Input: part model. Units: mm. Frame: model coordinates. Face numbers are marked on the shaded views. A direction names the side the tool comes from. Give positions to 0.01 mm unless a question says otherwise; leave off trailing zeros. Order: outer loops, then holes, each group sorted by start corner. A loop starts at its lowest first (then second) coordinate and runs counter-clockwise, first axis right, second up. Notation, with made-up numbers: M 67,74 L 109,74 A15 cw 109,101 Z; hole C -22.5,-15.75 d10. An arc over 180 degrees is marked long. Use a Markdown table: item, result.
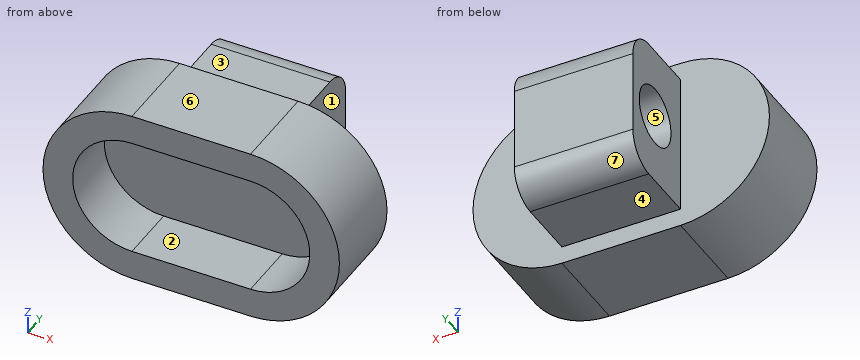
from build123d import *

# Parameters (mm, degrees)
F1_DEPTH = 15
F3_DEPTH = 5
F4_W     = 20
F4_H     = 24
F5_DEPTH = 15
F6_R     = 5
F7_R     = 5
F8_DEPTH = 25


with BuildPart() as f1:
    # F0 (on Front) → F1 (new body)
    with BuildSketch(Plane.XZ):
        with BuildLine():
            Line((-10, -15), (10, -15))
            ThreePointArc((10, -15), (25, 0), (10, 15))
            Line((10, 15), (-10, 15))
            ThreePointArc((-10, 15), (-25, 0), (-10, -15))
        make_face()
        with BuildLine():
            ThreePointArc((-10, -10), (-20, 0), (-10, 10))
            Line((-10, 10), (10, 10))
            ThreePointArc((10, 10), (20, 0), (10, -10))
            Line((10, -10), (-10, -10))
        make_face(mode=Mode.SUBTRACT)
    extrude(amount=F1_DEPTH)

    # F2 (on face) → F3 (join)
    with BuildSketch(Plane(origin=(0, 0, 0), x_dir=(-1, 0, 0), z_dir=(0, 1, 0))):
        with BuildLine():
            ThreePointArc((10, -10), (20, 0), (10, 10))
            Line((10, 10), (-10, 10))
            ThreePointArc((-10, 10), (-20, 0), (-10, -10))
            Line((-10, -10), (10, -10))
        make_face()
    extrude(amount=-F3_DEPTH)

    # F4 (on face) → F5 (join)
    with BuildSketch(Plane(origin=(0, 0, 0), x_dir=(-1, 0, 0), z_dir=(0, 1, 0))):
        Rectangle(F4_W, F4_H)
    extrude(amount=F5_DEPTH)

    # F6
    f6_edges = [f1.edges().sort_by_distance(p)[0] for p in [
        (0, 15, -12),
        (0, 15, 12),
    ]]
    fillet(f6_edges, radius=F6_R)

    # F7 (on face) → F8 (cut)
    with BuildSketch(Plane.YZ.offset(10)):
        with Locations((8, 0)):
            Circle(F7_R)
    extrude(amount=-F8_DEPTH, mode=Mode.SUBTRACT)


solid = f1.part
1) Cut plane D-D on x = 11.5. Return loops of the section in (y, z), and give its area (3 significant figures).
Response values:
| item | result |
|---|---|
| outline | M -15,-14.92 L 0,-14.92 L 0,14.92 L -15,14.92 L -15,9.89 L -5,9.89 L -5,-9.89 L -15,-9.89 Z |
| area | 250 mm² |
2) Mould query, pull axis Y, two halves, no side actions, for the marked faces 5, 6 and 7. Classes: released by +Y, released by -Y, zero draft, split by the parting line, or undercut.
Response values:
| item | result |
|---|---|
| face 5 | undercut |
| face 6 | zero draft |
| face 7 | released by +Y |
3) Cut plane C-C on x = 5.5. Return loops of the section in (y, z), and give its area (3 significant figures).
Response values:
| item | result |
|---|---|
| outline | M -15,-15 L 0,-15 L 0,-12 L 10,-12 A5 ccw 15,-7 L 15,7 A5 ccw 10,12 L 0,12 L 0,15 L -15,15 L -15,10 L -5,10 L -5,-10 L -15,-10 Z; hole C 8,0 d10 |
| area | 521 mm² |
4) Reachability of the marked faces 1, 2, 3 and 4 from +Z, -Z, +X, -X, +Y, -Y: full face, straight path, thin tool, end or side. Return the list, or none.
Response values:
| item | result |
|---|---|
| face 1 | +Z, -Z, +X, +Y |
| face 2 | -Y |
| face 3 | +Z, +X, -X, +Y |
| face 4 | -Z, +X, -X, +Y |
5) First-contact query: pin 1 Ø2 at (x, z) = (17, -5) entering from +Y; pin 2 Ø8 at (x, y) = (1, 5.5) entering from -Z; pin 3 Ø4 at (y, z) = (9, -6.5) entering from +X; pin 4 Ø11 at (x, y) = (-2, 3) entering from +Z. Flat tips, straight axial feed; report the tip coordinate or a pass-through.
Response values:
| item | result |
|---|---|
| pin 1 | stops at y = 0 |
| pin 2 | stops at z = -12 |
| pin 3 | stops at x = 10 |
| pin 4 | stops at z = 15 |
6) Cut plane A-A on z = 0. Return loops of the section in (x, y).
Response values:
| item | result |
|---|---|
| outline | M -25,-15 L -20,-15 L -20,-5 L 20,-5 L 20,-15 L 25,-15 L 25,0 L 10,0 L 10,3 L -10,3 L -10,0 L -25,0 Z; M -10,13 L 10,13 L 10,15 L -10,15 Z |
7) Material intervals for line 1 (Z direction, x = 4.5, y = 8); line 2 (Z direction, x = -0.5, y = -6.75); line 3 (X direction, y = -11.75, z = 0.5), sorted ascending. Write a range as from..to.
Response values:
| item | result |
|---|---|
| line 1 | z = -12..-5, 5..12 |
| line 2 | z = -15..-10, 10..15 |
| line 3 | x = -24.99..-19.99, 19.99..24.99 |
8) Cut plane B-B on y = 5.75. Return loops of the section in (x, z), and give its area (3 significant figures).
Response values:
| item | result |
|---|---|
| outline | M -10,-12 L 10,-12 L 10,-4.47 L -10,-4.47 Z; M -10,4.47 L 10,4.47 L 10,12 L -10,12 Z |
| area | 301 mm² |
